```python
from build123d import *

# Parameters (mm, degrees)
F2_DEPTH = 9.5
F3_T     = -0.8
F4_R     = 5
F5_SIZE  = 2
F0_R     = 1.5
F6_DEPTH = 2
F7_SIZE  = 1


with BuildPart() as f2:
    # F1 (on Front) → F2 (new body, symmetric)
    with BuildSketch(Plane.XZ):
        Polygon((-24, 0), (27.5, 0), (41, 20), (36, 20), (32.49, 14.8), (-24, 14.8), align=None)
    extrude(amount=F2_DEPTH, both=True)

    # F3
    f3_openings = [f2.faces().sort_by_distance(p)[0] for p in [
        (-24, 0, 7.4),
        (38.5, 0, 20),
    ]]
    offset(amount=F3_T, openings=f3_openings, kind=Kind.INTERSECTION)

    # F4
    f4_edges = [f2.edges().sort_by_distance(p)[0] for p in [
        (27.074806, 0, 0.8),
    ]]
    fillet(f4_edges, radius=F4_R)

    # F5
    f5_edges = [f2.edges().sort_by_distance(p)[0] for p in [
        (4.457597, -8.7, 14),
        (4.457597, 8.7, 14),
        (0.208671, 8.7, 0.8),
        (0.208671, -8.7, 0.8),
        (26.763954, 8.7, 1.384866),
        (34.298195, 8.7, 11.501318),
        (26.763954, -8.7, 1.384866),
        (34.298195, -8.7, 11.501318),
    ]]
    chamfer(f5_edges, length=F5_SIZE)

    # F0 (on Top) → F6 (join)
    with BuildSketch(Plane.XY):
        with BuildLine():
            Line((2.5, -9.5), (-4.5, -9.5))
            Line((-4.5, -9.5), (-4.5, -13))
            ThreePointArc((-4.5, -13), (-1.2506305341, -17.0266392409), (2.5355339059, -13.5))
            Line((2.5355339059, -13.5), (2.5355339059, -9.5))
            Line((2.5355339059, -9.5), (2.5, -9.5))
        make_face()
        with Locations((-1, -13.5)):
            Circle(F0_R, mode=Mode.SUBTRACT)
        with BuildLine():
            Line((-4.5, 13), (-4.5, 9.5))
            Line((-4.5, 9.5), (2.5, 9.5))
            Line((2.5, 9.5), (2.5355339059, 9.5))
            Line((2.5355339059, 9.5), (2.5355339059, 13.5))
            ThreePointArc((2.5355339059, 13.5), (-1.2506305341, 17.0266392409), (-4.5, 13))
        make_face()
        with Locations((-1, 13.5)):
            Circle(F0_R, mode=Mode.SUBTRACT)
    extrude(amount=F6_DEPTH)

    # F7
    f7_edges = [f2.edges().sort_by_distance(p)[0] for p in [
        (34.25, 9.5, 10),
        (34.25, -9.5, 10),
    ]]
    chamfer(f7_edges, length=F7_SIZE)


solid = f2.part
```
CAD build for the part. Positions are in the model's coordinates, mm. A direction names the side the tool comes from. Round coordinates to 2 decimals unless told otherwise and drop trailing zeros. Order: outer loops, then holes, each group sorted by start corner. A loop starts at its lowest first (then second) coordinate and runs counter-clockwise, first axis right, second up. Notation, with made-up numbers: (-40, 86.25) - (-3, 86.25) arc R11 cw to (-3, 90.25) - close; hole circle Ø9 at (22.5, -15). An arc over 180 degrees is marked (long way). Use CSV: the item, a comma, the result in double quotes. Start each with the question number.
1) Wall check: L1, parallel to Y at x = -1, z = 0.7; L2, parallel to Y at x = 6.5, z = 8.75; L3, parallel to Z at x = -21, y = 4.5. Give the ranges that are in metal, low to high. Write a range as [from, to].
2) Pin check, flat tips, straight feed: pin 1 Ø0.6 at (y, z) = (-12, 1) entering from +X; pin 2 Ø4 at (x, y) = (31, -10.5) entering from -Z; pin 3 Ø5 at (y, z) = (-1.5, 7.5) entering from +X; pin 4 Ø2.5 at (x, y) = (-1, 13.5) entering from -Z. Stop position of each tip, or through.
3) Two-plate mould, pull along Y, no slides. Class faces 1 (the flat face through (1, 0, 0)), 2 (the cylindrical face through (-2.2, 12.6, 1)), 3 (the flat face through (33.56, -8.99, 9.85)), 4 (the flat face through (33.56, 8.99, 9.85)): pulls with the +Y half, pulls with the -Y half, needs draft (parallel to the pull), parting line crosses it, or undercut.
4) Saw through at D-D (z = 5.5). List the corners of the cut face in (x, y).
5) Saw through at A-A (x = -1). List the corners of the cut face in (y, z).
6) Tool access for faces 5 (the flat face through (0, 0, 0.8)), 6 (the flat face through (-1, -11.5, 2)), 7 (the flat face through (34.9, -0.12, 16.94)), 8 (the flat face through (-1, 11.6, 2)): list every direction of +Z, -Z, +X, -X, +Y, -Y with a clear straight run to the whole face (end or side of a thin tool).
7) Saw through at C-C (x = 17.5). List the corners of the cut face in (y, z).
8) Saw through at B-B (y = -6). List the corners of the cut face in (x, z), and give its area (3 significant figures).
Values follow:
1,L1,"y = [-17.04, -15], [-12, 12], [15, 17.04]"
1,L2,"y = [-9.5, -8.7], [8.7, 9.5]"
1,L3,"z = [0, 0.8], [14, 14.8]"
2,pin 1,"stops at x = 2.54"
2,pin 2,"stops at z = 4.12"
2,pin 3,"stops at x = 34.25"
2,pin 4,"passes through"
3,face 1,"needs draft"
3,face 2,"undercut"
3,face 3,"pulls with the -Y half"
3,face 4,"pulls with the +Y half"
4,outline,"(-24, -9.5) - (30.01, -9.5) - (31.21, -8.5) - (31.21, 8.5) - (30.01, 9.5) - (-24, 9.5) - (-24, 8.7) - (27.83, 8.7) - (30.25, 6.7) - (30.25, -6.7) - (27.83, -8.7) - (-24, -8.7) - close"
5,outline,"(-17.04, 0) - (-15, 0) - (-15, 2) - (-17.04, 2) - close; (-12, 0) - (12, 0) - (12, 2) - (9.5, 2) - (9.5, 14.8) - (-9.5, 14.8) - (-9.5, 2) - (-12, 2) - close; (15, 0) - (17.04, 0) - (17.04, 2) - (15, 2) - close; hole (-8.7, 2.8) - (-6.7, 0.8) - (6.7, 0.8) - (8.7, 2.8) - (8.7, 12) - (6.7, 14) - (-6.7, 14) - (-8.7, 12) - close"
6,face 5,"-X"
6,face 6,"+Z, +X, -X, -Y"
6,face 7,"none"
6,face 8,"+Z, +X, -X, +Y"
7,outline,"(-9.5, 0) - (9.5, 0) - (9.5, 14.8) - (-9.5, 14.8) - close; hole (-8.7, 2.8) - (-6.7, 0.8) - (6.7, 0.8) - (8.7, 2.8) - (8.7, 12) - (6.7, 14) - (-6.7, 14) - (-8.7, 12) - close"
8,outline,"(-24, 0) - (27.5, 0) - (41, 20) - (40.03, 20) - (28.56, 3) arc R5 cw to (24.42, 0.8) - (-24, 0.8) - close; (-24, 14) - (32.92, 14) - (36.97, 20) - (36, 20) - (32.49, 14.8) - (-24, 14.8) - close"
8,area,"112 mm2"
